Source: CAD feature listing. Evaluate the final solid. Frame: model axes, mm. A direction names the side the tool comes from. Round coordinates to 2 decimals unless told otherwise and drop trailing zeros. Order: outer loops, then holes, each group sorted by start corner. A loop starts at its lowest first (then second) coordinate and runs counter-clockwise, first axis right, second up. Notation, with made-up numbers: (-1, 11.25) - (24, 11.25) arc R15 cw to (24, 22.25) - close; hole circle Ø5 at (22.25, 38). An arc over 180 degrees is marked (long way). Return JSON: item names as keys, results as strings. Group by question number.
1) Section B-B, the plane z = 102. Return loops of the section in (x, y).
2) Section A-A, the plane y = -5.5. Return loops of the section in (x, z), plus the area to 3 significant figures.
3) Mould query, pull axis Z, two halves, no side actions, for faces 4 (the cylindrical face through (118, -8, 119)), 5 (the cylindrical face through (2.86, -7.6, 117.1)), 6 (the cylindrical face through (1, -18, 61)). Classes: pulls with the +Z half, pulls with the -Z half, needs draft (parallel to the pull), parting line crosses it, or undercut.
4) Ray query, line 1 (Z direction, x = 60, y = -9.5); line 2 (Z direction, x = 60, y = -29); line 3 (X direction, y = -5.5, z = 9). Return the intervals inside material, ascending. Write a range as from..to.
5) Contact query for flat-ended pins moving along their axis: P1, Ø10, axis at x = 43, z = 33.5, coming from the +Y side; P2, Ø2, axis at x = 59, y = -18, coming from the +Z side; P3, Ø3, axis at x = 37.5, y = -28, coming from the -Z side; P4, Ø1, axis at x = 97, z = 96, coming from the -Y side. Output: stop coordinate, or through.
6) Access query for faces 1 (the cylindrical face through (2.86, -17.1, 60.77)), 2 (the cylindrical face through (61, -18, 1)), 3 (the flat face through (35, -20, 97)). Directions: +Z, -Z, +X, -X, +Y, -Y. A direction counts if a zero-diameter tool reaches every point of the face in a straight line with its end or side. Return the directions, or none.
7) Section D-D, the plane y = -30. Return loops of the section in (x, z).
8) Section C-C, the plane x = 103. Return loops of the section in (y, z), plus the area to 3 significant figures.
```python
from build123d import *

# Parameters (mm, degrees)
F4_W     = 120
F4_H     = 120
F0_DEPTH = 20
F5_R     = 35
F1_DEPTH = 15
F2_R     = 25
F6_DEPTH = 35
F3_R     = 5
F7_R     = 1.5
F8_T     = -2


with BuildPart() as f0:
    # F4 (on Front) → F0 (new body)
    with BuildSketch(Plane.XZ):
        with Locations((60, 60)):
            Rectangle(F4_W, F4_H)
    extrude(amount=F0_DEPTH)

    # F5 (on face) → F1 (join)
    with BuildSketch(Plane.XZ.offset(20)):
        with Locations((60, 60)):
            Circle(F5_R)
    extrude(amount=F1_DEPTH)

    # F2 (on face) → F6 (cut, through all)
    with BuildSketch(Plane.XZ.offset(35)):
        with Locations((60, 60)):
            Circle(F2_R)
    extrude(amount=-F6_DEPTH, mode=Mode.SUBTRACT)

    # F3
    f3_edges = [f0.edges().sort_by_distance(p)[0] for p in [
        (120, -10, 120),
        (60, -20, 120),
        (120, -20, 60),
        (60, -20, 0),
        (0, -20, 60),
        (0, -10, 120),
        (0, -10, 0),
        (120, -10, 0),
        (25, -20, 60),
    ]]
    fillet(f3_edges, radius=F3_R)

    # F7
    f7_edges = [f0.edges().sort_by_distance(p)[0] for p in [
        (25, -35, 60),
        (35, -35, 60),
    ]]
    fillet(f7_edges, radius=F7_R)

    # F8
    f8_openings = [f0.faces().sort_by_distance(p)[0] for p in [
        (1.697056, 0, 60),
    ]]
    offset(amount=F8_T, openings=f8_openings)


solid = f0.part
```
Geometry check:
{
 "1": {"outline": "(0, -15) arc R5 ccw to (5, -20) - (115, -20) arc R5 ccw to (120, -15) - (120, 0) - (118, 0) - (118, -15) arc R3 cw to (115, -18) - (5, -18) arc R3 cw to (2, -15) - (2, 0) - (0, 0) - close"},
 "2": {"outline": "(0, 5) arc R5 ccw to (5, 0) - (115, 0) arc R5 ccw to (120, 5) - (120, 115) arc R5 ccw to (115, 120) - (5, 120) arc R5 ccw to (0, 115) - close; circle Ø54 at (60, 60); hole (2, 5) arc R3 ccw to (5, 2) - (115, 2) arc R3 ccw to (118, 5) - (118, 115) arc R3 ccw to (115, 118) - (5, 118) arc R3 ccw to (2, 115) - close; hole circle Ø50 at (60, 60)", "area": "1,260 mm2"},
 "3": {"face 4": "pulls with the +Z half", "face 5": "undercut", "face 6": "needs draft"},
 "4": {"line 1": "0..2, 33..35, 85..87, 118..120", "line 2": "25..27, 33..35, 85..87, 93..95", "line 3": "0..2, 118..120"},
 "5": {"P1": "y = 0", "P2": "z = 119.58", "P3": "z = 32", "P4": "y = -20"},
 "6": {"face 1": "+Y", "face 2": "-Z, +X, -X, -Y", "face 3": "-Y"},
 "7": {"outline": "circle Ø70 at (60, 60); circle Ø54 at (60, 60); hole circle Ø66 at (60, 60); hole circle Ø50 at (60, 60)"},
 "8": {"outline": "(-20, 5) arc R5 ccw to (-15, 0) - (0, 0) - (0, 2) - (-15, 2) arc R3 cw to (-18, 5) - (-18, 115) arc R3 cw to (-15, 118) - (0, 118) - (0, 120) - (-15, 120) arc R5 ccw to (-20, 115) - close", "area": "305 mm2"}
}
